Input: part model. Units: mm. Frame: model coordinates. Face numbers are marked on the shaded views. Coordinates: 2 decimals unless noted, no trailing zeros. Order: outer loops, then holes, each group sorted by start corner. A loop starts at its lowest first (then second) coordinate and runs counter-clockwise, first axis right, second up. Notation, with made-up numbers: (-17, 37) -> (13, 37) arc R27 ccw to (13, 72) -> close; hole circle Ø3 at (-7, 1.5). An arc over 180 degrees is marked (long way). Answer as CSV lines item,"result".
from build123d import *

# Parameters (mm, degrees)
SKETCH_1_W          = 40
SKETCH_1_H          = 39.9
EXTRUDE_1_DEPTH     = 2
SKETCH_2_R          = 1.45
CUT_EXTRUDE_1_DEPTH = 2
CUT_EXTRUDE_3_REACH = 58.533
SKETCH_5_R          = 1.45
SKETCH_7_W          = 6.4
SKETCH_7_H          = 39.9
CUT_EXTRUDE_5_DEPTH = 0.8


with BuildPart() as part:
    # 草图1 → 凸台-拉伸1 (new body)
    with BuildSketch(Plane(origin=(0, 0, 0), x_dir=(1, 0, 0), z_dir=(0, 1, 0))):
        with Locations((20, 19.95)):
            Rectangle(SKETCH_1_W, SKETCH_1_H)
    extrude(amount=EXTRUDE_1_DEPTH)

    # 草图2 → 切除-拉伸1 (cut)
    with BuildSketch(Plane(origin=(0, 2, 0), x_dir=(1, 0, 0), z_dir=(0, 1, 0))):
        with Locations(Location((2.5, 11.95, 0), (0, 0, 270))):
            Circle(SKETCH_2_R)
        with Locations(Location((17.5, 11.95, 0), (0, 0, 270))):
            Circle(SKETCH_2_R)
        with Locations(Location((17.5, 27.95, 0), (0, 0, 270))):
            Circle(SKETCH_2_R)
        with Locations(Location((2.5, 27.95, 0), (0, 0, 270))):
            Circle(SKETCH_2_R)
    extrude(amount=-CUT_EXTRUDE_1_DEPTH, mode=Mode.SUBTRACT)

    # 草图5 → 切除-拉伸3 (cut, up to next)
    with BuildSketch(Plane.XZ, mode=Mode.PRIVATE) as cut_extrude_3_sk1:
        with Locations(Location((22.25, -10, 0), (0, 0, 270))):
            Circle(SKETCH_5_R)
    cut_extrude_3_tool1 = extrude(cut_extrude_3_sk1.sketch, amount=-CUT_EXTRUDE_3_REACH, mode=Mode.PRIVATE) & part.part
    # 草图5 → 切除-拉伸3 (cut, up to next)
    with BuildSketch(Plane.XZ, mode=Mode.PRIVATE) as cut_extrude_3_sk2:
        with Locations(Location((36, -10, 0), (0, 0, 270))):
            Circle(SKETCH_5_R)
    cut_extrude_3_tool2 = extrude(cut_extrude_3_sk2.sketch, amount=-CUT_EXTRUDE_3_REACH, mode=Mode.PRIVATE) & part.part
    # 草图5 → 切除-拉伸3 (cut, up to next)
    with BuildSketch(Plane.XZ, mode=Mode.PRIVATE) as cut_extrude_3_sk3:
        with Locations(Location((36, -29.9, 0), (0, 0, 270))):
            Circle(SKETCH_5_R)
    cut_extrude_3_tool3 = extrude(cut_extrude_3_sk3.sketch, amount=-CUT_EXTRUDE_3_REACH, mode=Mode.PRIVATE) & part.part
    # 草图5 → 切除-拉伸3 (cut, up to next)
    with BuildSketch(Plane.XZ, mode=Mode.PRIVATE) as cut_extrude_3_sk4:
        with Locations(Location((22.25, -29.9, 0), (0, 0, 270))):
            Circle(SKETCH_5_R)
    cut_extrude_3_tool4 = extrude(cut_extrude_3_sk4.sketch, amount=-CUT_EXTRUDE_3_REACH, mode=Mode.PRIVATE) & part.part
    add(cut_extrude_3_tool1.solids().sort_by_distance((22.25, 0, -10))[0], mode=Mode.SUBTRACT)
    add(cut_extrude_3_tool2.solids().sort_by_distance((36, 0, -10))[0], mode=Mode.SUBTRACT)
    add(cut_extrude_3_tool3.solids().sort_by_distance((36, 0, -29.9))[0], mode=Mode.SUBTRACT)
    add(cut_extrude_3_tool4.solids().sort_by_distance((22.25, 0, -29.9))[0], mode=Mode.SUBTRACT)

    # 草图7 → 切除-拉伸5 (cut)
    with BuildSketch(Plane.XZ):
        with Locations((27.5, -19.95)):
            Rectangle(SKETCH_7_W, SKETCH_7_H)
    extrude(amount=-CUT_EXTRUDE_5_DEPTH, mode=Mode.SUBTRACT)


solid = part.part
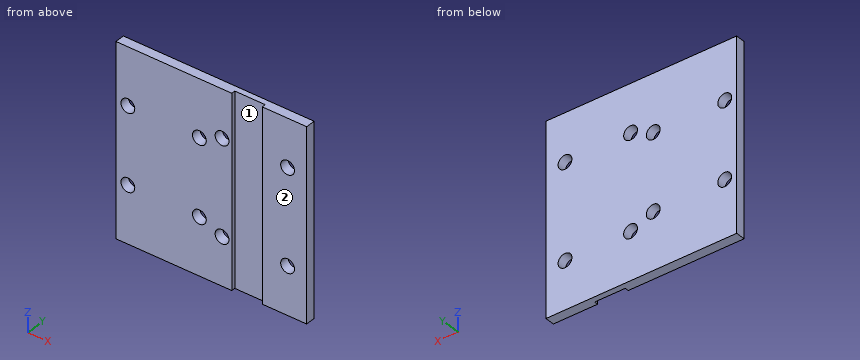
1. Ray query, line 1 along X through (y, z) = (0.9, -30); line 2 along X through (y, z) = (1.6, -27.95); line 3 along X through (y, z) = (0.2, -36.5). Return the intervals inside material, ascending.
Findings:
line 1,"x = 0 to 20.8, 23.7 to 34.55, 37.45 to 40"
line 2,"x = 0 to 1.05, 3.95 to 16.05, 18.95 to 40"
line 3,"x = 0 to 24.3, 30.7 to 40"
2. Cut plane B-B (x = 17.5). Return the cut outline in (y, z).
Findings:
outline,"(0, -39.9) -> (2, -39.9) -> (2, -29.4) -> (0, -29.4) -> close; (0, -26.5) -> (2, -26.5) -> (2, -13.4) -> (0, -13.4) -> close; (0, -10.5) -> (2, -10.5) -> (2, 0) -> (0, 0) -> close"
3. Mould query, pull axis X, two halves, no side actions, for the marked faces 1 and 2. Classes: released by +X, released by -X, zero draft, split by the parting line, or undercut.
Findings:
face 1,"undercut"
face 2,"zero draft"
4. Cut plane A-A (y = 0.5). State how many separate pieces and enclosed holes the cut face has, plus the area to 3 significant figures.
Findings:
separate pieces,"2"
enclosed holes,"8"
area,"1,290 mm2"
5. Contact query for flat-ended pins moving along their axis: pin 1 (1.9 mm diameter, centred on x = 27, z = -18, fed in from -Y); pin 2 (2.5 mm diameter, centred on x = 22.25, z = -10, fed in from -Y). Output: stop coordinate, or through.
Findings:
pin 1,"stops at y = 0.8"
pin 2,"passes through"
6. Cut plane D-D (x = 23). Return the cut outline in (y, z), plus the area to 3 significant figures.
Findings:
outline,"(0, -39.9) -> (2, -39.9) -> (2, -31.14) -> (0, -31.14) -> close; (0, -28.66) -> (2, -28.66) -> (2, -11.24) -> (0, -11.24) -> close; (0, -8.76) -> (2, -8.76) -> (2, 0) -> (0, 0) -> close"
area,"69.9 mm2"
7. Cut plane C-C (z = -10). Return the cut outline in (x, y), plus the area to 3 significant figures.
Findings:
outline,"(0, 0) -> (20.8, 0) -> (20.8, 2) -> (0, 2) -> close; (23.7, 0) -> (24.3, 0) -> (24.3, 0.8) -> (30.7, 0.8) -> (30.7, 0) -> (34.55, 0) -> (34.55, 2) -> (23.7, 2) -> close; (37.45, 0) -> (40, 0) -> (40, 2) -> (37.45, 2) -> close"
area,"63.3 mm2"
